```python
from build123d import *

# Parameters (mm, degrees)
F1_DEPTH = 30.12
F3_DEPTH = 55.26
F6_DEPTH = 7.5
F8_DEPTH = 1.5
F9_DEPTH = 13.7
F10_R    = 3


with BuildPart() as f1:
    # F0 (on Right) → F1 (new body)
    with BuildSketch(Plane.YZ):
        with BuildLine():
            ThreePointArc((0, -7.395), (5.2290546469, -5.2290546469), (7.395, 0))
            ThreePointArc((7.395, 0), (5.2290546469, 5.2290546469), (0, 7.395))
            Line((0, 7.395), (-0.1808295417, 7.3927887618))
            ThreePointArc((-0.1808295417, 7.3927887618), (-5.2926014143, 5.1647260595), (-7.395, 0))
            Line((-7.395, 0), (-7.3927887618, -0.1808295417))
            ThreePointArc((-7.3927887618, -0.1808295417), (-5.1647260595, -5.2926014143), (0, -7.395))
        make_face()
        Polygon((-4.2, 1.7), (-4.2, 4.5), (4.2, 4.5), (4.2, -4.5), (-4.2, -4.5), (-4.2, -1.7), (-6.1, -1.7), (-6.1, 1.7), align=None, mode=Mode.SUBTRACT)
        with BuildLine():
            Line((-7.3045717093, -7.395), (0, -7.395))
            ThreePointArc((0, -7.395), (-5.1647260595, -5.2926014143), (-7.3927887618, -0.1808295417))
            Line((-7.3927887618, -0.1808295417), (-7.3045717093, -7.395))
        make_face()
        with BuildLine():
            ThreePointArc((-7.395, 0), (-5.2926014143, 5.1647260595), (-0.1808295417, 7.3927887618))
            Line((-0.1808295417, 7.3927887618), (-7.4843091518, 7.3034796101))
            Line((-7.4843091518, 7.3034796101), (-7.395, 0))
        make_face()
        with BuildLine():
            Line((7.395, -7.395), (7.395, 0))
            ThreePointArc((7.395, 0), (5.2290546469, -5.2290546469), (0, -7.395))
            Line((0, -7.395), (7.395, -7.395))
        make_face()
        with BuildLine():
            ThreePointArc((0, 7.395), (5.2290546469, 5.2290546469), (7.395, 0))
            Line((7.395, 0), (7.395, 7.395))
            Line((7.395, 7.395), (0, 7.395))
        make_face()
    extrude(amount=F1_DEPTH)

    # F2 (on face) → F3 (join)
    with BuildSketch(Plane.YZ.offset(30.12)):
        with BuildLine():
            ThreePointArc((-7.395, 0), (-5.2926014143, 5.1647260595), (-0.1808295417, 7.3927887618))
            Line((-0.1808295417, 7.3927887618), (-7.4843091518, 7.3034796101))
            Line((-7.4843091518, 7.3034796101), (-7.395, 0))
        make_face()
        with BuildLine():
            Line((2.9646117869, 4.5), (2.9646117869, 6.7747399916))
            ThreePointArc((2.9646117869, 6.7747399916), (1.5144013277, 7.2382742155), (0, 7.395))
            Line((0, 7.395), (-0.1808295417, 7.3927887618))
            ThreePointArc((-0.1808295417, 7.3927887618), (-5.2926014143, 5.1647260595), (-7.395, 0))
            Line((-7.395, 0), (-7.3927887618, -0.1808295417))
            ThreePointArc((-7.3927887618, -0.1808295417), (-5.1647260595, -5.2926014143), (0, -7.395))
            ThreePointArc((0, -7.395), (1.5144013277, -7.2382742155), (2.9646117869, -6.7747399916))
            Line((2.9646117869, -6.7747399916), (2.9646117869, -4.5))
            Line((2.9646117869, -4.5), (-4.2, -4.5))
            Line((-4.2, -4.5), (-6.1, -1.7))
            Line((-6.1, -1.7), (-6.1, 1.7))
            Line((-6.1, 1.7), (-4.2, 4.5))
            Line((-4.2, 4.5), (2.9646117869, 4.5))
        make_face()
        with BuildLine():
            Line((-7.3045717093, -7.395), (0, -7.395))
            ThreePointArc((0, -7.395), (-5.1647260595, -5.2926014143), (-7.3927887618, -0.1808295417))
            Line((-7.3927887618, -0.1808295417), (-7.3045717093, -7.395))
        make_face()
    extrude(amount=F3_DEPTH)

    # F5 (on Front) → F6 (join, symmetric)
    with BuildSketch(Plane.XZ):
        with BuildLine():
            Line((93.34, 7.395), (85.38, 7.395))
            Line((85.38, 7.395), (85.38, -7.395))
            Line((85.38, -7.395), (93.34, -7.395))
            ThreePointArc((93.34, -7.395), (89.43, 0), (93.34, 7.395))
        make_face()
    extrude(amount=F6_DEPTH, both=True)

    # F7 (on Front) → F8 (join, symmetric)
    with BuildSketch(Plane.XZ):
        with BuildLine():
            add(Edge.make_bspline(
                [(99.5611976313, -6.9222719045), (97.6347457755, -7.5906937073), (93.8964104218, -8.4654582573), (90.4010751726, -7.8833055428), (88.7074694037, -7.395)],
                knots=[0, 0, 0, 0, 0.5144212355, 1, 1, 1, 1], degree=3))
            add(Edge.make_bspline(
                [(99.5611976313, -6.9222719045), (97.217178841, -7.58868722), (94.1584374095, -7.2106656851), (93.34, -7.395)],
                knots=[3.9877929831, 3.9877929831, 3.9877929831, 3.9877929831, 9.8433615853, 9.8433615853, 9.8433615853, 9.8433615853], degree=3))
            Line((93.34, -7.395), (88.7074694037, -7.395))
        make_face()
        with BuildLine():
            add(Edge.make_bspline(
                [(99.5611976313, -6.9222719045), (97.217178841, -7.58868722), (94.1584374095, -7.2106656851), (93.34, -7.395)],
                knots=[3.9877929831, 3.9877929831, 3.9877929831, 3.9877929831, 9.8433615853, 9.8433615853, 9.8433615853, 9.8433615853], degree=3))
            add(Edge.make_bspline(
                [(102.4147021825, -3.8559928472), (102.3072303482, -5.6141000369), (101.0852953963, -6.488963905), (99.5611976313, -6.9222719045)],
                knots=[0.1804604412, 0.1804604412, 0.1804604412, 0.1804604412, 3.9877929831, 3.9877929831, 3.9877929831, 3.9877929831], degree=3))
            add(Edge.make_bspline(
                [(102.4147021825, -3.8559928472), (101.0774964274, -4.8978899586), (99.4699665658, -5.3518592672), (98.3198470269, -5.449623214), (93.894019065, -5.2308255551), (93.3923863769, 0)],
                knots=[0.0006270435, 0.0006270435, 0.0006270435, 0.0006270435, 0.3281259648, 0.5118184212, 1, 1, 1, 1], degree=3))
            add(Edge.make_bspline(
                [(102.4147021825, 3.8559928472), (101.0774964274, 4.8978899586), (99.4699665658, 5.3518592672), (98.3198470269, 5.449623214), (93.894019065, 5.2308255551), (93.3923863769, 0)],
                knots=[0.0006270435, 0.0006270435, 0.0006270435, 0.0006270435, 0.3281259648, 0.5118184212, 1, 1, 1, 1], degree=3))
            add(Edge.make_bspline(
                [(102.4147021825, 3.8559928472), (102.3072303482, 5.6141000369), (101.0852953963, 6.488963905), (99.5611976313, 6.9222719045)],
                knots=[0.1804604412, 0.1804604412, 0.1804604412, 0.1804604412, 3.9877929831, 3.9877929831, 3.9877929831, 3.9877929831], degree=3))
            add(Edge.make_bspline(
                [(99.5611976313, 6.9222719045), (97.217178841, 7.58868722), (94.1584374095, 7.2106656851), (93.34, 7.395)],
                knots=[3.9877929831, 3.9877929831, 3.9877929831, 3.9877929831, 9.8433615853, 9.8433615853, 9.8433615853, 9.8433615853], degree=3))
            ThreePointArc((93.34, 7.395), (89.43, 0), (93.34, -7.395))
        make_face()
        with BuildLine():
            Line((88.7074694037, 7.395), (93.34, 7.395))
            add(Edge.make_bspline(
                [(99.5611976313, 6.9222719045), (97.217178841, 7.58868722), (94.1584374095, 7.2106656851), (93.34, 7.395)],
                knots=[3.9877929831, 3.9877929831, 3.9877929831, 3.9877929831, 9.8433615853, 9.8433615853, 9.8433615853, 9.8433615853], degree=3))
            add(Edge.make_bspline(
                [(99.5611976313, 6.9222719045), (97.6347457755, 7.5906937073), (93.8964104218, 8.4654582573), (90.4010751726, 7.8833055428), (88.7074694037, 7.395)],
                knots=[0, 0, 0, 0, 0.5144212355, 1, 1, 1, 1], degree=3))
        make_face()
    extrude(amount=F8_DEPTH, both=True)

    # F4 (on face) → F9 (cut)
    with BuildSketch(Plane.YZ.offset(85.38)):
        with BuildLine():
            Line((-8.1289913505, 8.4002688527), (-8.1289913505, -8.4002688527))
            Line((-8.1289913505, -8.4002688527), (2.9646117869, -8.4002688527))
            Line((2.9646117869, -8.4002688527), (2.9646117869, -6.7747399916))
            ThreePointArc((2.9646117869, -6.7747399916), (1.5144013277, -7.2382742155), (0, -7.395))
            Line((0, -7.395), (-7.3045717093, -7.395))
            Line((-7.3045717093, -7.395), (-7.4843091518, 7.3034796101))
            Line((-7.4843091518, 7.3034796101), (0, 7.395))
            ThreePointArc((0, 7.395), (1.5144013277, 7.2382742155), (2.9646117869, 6.7747399916))
            Line((2.9646117869, 6.7747399916), (2.9646117869, 8.4002688527))
            Line((2.9646117869, 8.4002688527), (-8.1289913505, 8.4002688527))
        make_face()
        Polygon((2.9646117869, -6.7747399916), (2.9646117869, -8.4002688527), (8.1289913505, -8.4002688527), (8.1289913505, 8.4002688527), (2.9646117869, 8.4002688527), (2.9646117869, 6.7747399916), (2.9646117869, 4.5), (2.9646117869, -4.5), align=None)
    extrude(amount=F9_DEPTH, mode=Mode.SUBTRACT)

    # F10
    f10_edges = [f1.edges().sort_by_distance(p)[0] for p in [
        (46.67, -7.304572, -7.395),
        (15.06, 7.395, 7.395),
        (15.06, 7.395, -7.395),
        (46.60411, -7.484309, 7.30348),
    ]]
    fillet(f10_edges, radius=F10_R)


solid = f1.part
```
Geometry check sheet. Reference: the model listing, model coordinates, mm. A direction names the side the tool comes from. Coordinates: 2 decimals unless noted, no trailing zeros. Write each loop counter-clockwise with the first axis right and the second up, starting at its lowest first coordinate (ties: lowest second). Pieces come first, ordered by that corner, then holes. Notation, with made-up numbers: M -19.5,-23 L -0.5,-23 A38 ccw -0.5,15 Z; hole C -22.75,0.5 d8. An arc over 180 degrees is marked long. Use one line per item in the form item = value. Start each with the question number.
1) Release check for a two-part mould opening along X. For faces 1 (the flat face through (30.12, 5, 0)), 2 (the flat face through (30.12, -5, 2)), 3 (the flat face through (93, -1.5, 0)) record: pulls with the +X half, pulls with the -X half, needs draft (parallel to the pull), parting line crosses it, or undercut.
2) Set-up check for faces 4 (the flat face through (15, 4.2, 0)), 5 (the flat face through (15, -4.2, -3)), 6 (the flat face through (68, 2.965, 5)), 7 (the cylindrical face through (63.874, 1.493, 7.243)), 8 (the cylindrical face through (89.43, 2.22, -0.12)): record each of +Z, -Z, +X, -X, +Y, -Y from which the full face is reachable in a straight line by a thin tool's end or side.
3) Thickness scan on probe 1 along Z at (x, y) = (35.5, -3) (3 decimals); probe 2 along Z at (x, y) = (41, -3.75) (3 decimals); probe 3 along Y at (x, z) = (10.5, 2.75) (3 decimals). Record the ranges inside material, lowest first. Write a range as from..to.
4) Go/stop test with flat-tipped pins: pin 1 Ø2 at (y, z) = (6, 2) entering from +X; pin 2 Ø3 at (x, z) = (68, 0.5) entering from +Y; pin 3 Ø0.9 at (y, z) = (-5, 2.5) entering from +X. Record where each tip stops, or that it passes through.
5) Section check A-A on x = 55.5. Enter the section's corners in (y, z) (3 decimals).
6) Section check B-B on x = 17. Enter the section's corners in (y, z) (3 decimals), and give its area (3 significant figures).
Responses:
q1.face_1 = pulls with the +X half
q1.face_2 = undercut
q1.face_3 = needs draft
q2.face_4 = +X, -X
q2.face_5 = -X
q2.face_6 = +Z, -Z, +X, +Y
q2.face_7 = +Z, +X, +Y
q2.face_8 = +X, +Y
q3.probe_1 = -7.395..-4.5, 4.5..7.358
q3.probe_2 = -7.395..-4.5, 4.5..7.349
q3.probe_3 = -7.429..-4.2, 4.2..7.395
q4.pin_1 = 30.12
q4.pin_2 = -5.9
q4.pin_3 = 89.93
q5.outline = M -7.448,4.304 L -7.341,-4.432 A3 ccw -4.341,-7.395 L 0,-7.395 A7.395 ccw 2.965,-6.775 L 2.965,-4.5 L -4.2,-4.5 L -6.1,-1.7 L -6.1,1.7 L -4.2,4.5 L 2.965,4.5 L 2.965,6.775 A7.395 ccw 0,7.395 L -4.485,7.34 A3 ccw Z
q6.outline = M -7.448,4.304 L -7.341,-4.432 A3 ccw -4.341,-7.395 L 4.395,-7.395 A3 ccw 7.395,-4.395 L 7.395,4.395 A3 ccw 4.395,7.395 L 0,7.395 L -4.485,7.34 A3 ccw Z; hole M -6.1,-1.7 L -4.2,-1.7 L -4.2,-4.5 L 4.2,-4.5 L 4.2,4.5 L -4.2,4.5 L -4.2,1.7 L -6.1,1.7 Z
q6.area = 129 mm2
